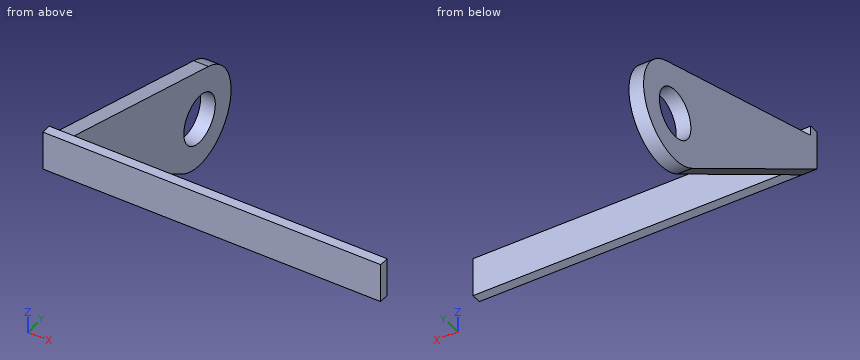
from build123d import *

# Parameters (mm, degrees)
SKETCH1_W           = 2.032
SKETCH1_H           = 0.508
BOSS_EXTRUDE1_DEPTH = 17.526
SKETCH1_3_R         = 2.54
SKETCH1_3_R_2       = 1.27
BOSS_EXTRUDE2_DEPTH = 0.762


with BuildPart() as part:
    # Sketch1 → Boss-Extrude1 (new body)
    with BuildSketch(Plane(origin=(0, 0, 0), x_dir=(0, 0, -1), z_dir=(1, 0, 0))):
        with Locations((-5.334, -11.176)):
            Rectangle(SKETCH1_W, SKETCH1_H)
    extrude(amount=BOSS_EXTRUDE1_DEPTH)

    # Sketch1_3 → Boss-Extrude2 (add)
    # profile 1 of 2: a face of its own
    with BuildSketch(Plane(origin=(0, 0, 0), x_dir=(0, 0, -1), z_dir=(1, 0, 0))):
        with BuildLine():
            Line((-4.318, -11.43), (2.137587014, -1.371977316))
            ThreePointArc((2.137587014, -1.371977316), (-1.053360752, -2.311283437), (-2.437803052, 0.713243493))
            Line((-2.437803052, 0.713243493), (-5.842, -10.922))
            Line((-5.842, -10.922), (-4.318, -10.922))
            Line((-4.318, -10.922), (-4.318, -11.43))
        make_face()
    # profile 2 of 2: a face of its own
    with BuildSketch(Plane(origin=(0, 0, 0), x_dir=(0, 0, -1), z_dir=(1, 0, 0))):
        Circle(SKETCH1_3_R)
        with Locations(Location((0, 0, 0), (0, 0, 180))):
            Circle(SKETCH1_3_R_2, mode=Mode.SUBTRACT)
    extrude(amount=BOSS_EXTRUDE2_DEPTH)


solid = part.part
Can you work these out from the model? Positions are in its coordinate system, mm. Round coordinates to 2 decimals unless told otherwise and drop trailing zeros. Order: outer loops, then holes, each group sorted by start corner. A loop starts at its lowest first (then second) coordinate and runs counter-clockwise, first axis right, second up. Notation, with made-up numbers: M -2.75,64 L 50.25,64 A7 ccw 50.25,74 Z; hole C 65.25,76.5 d7. An arc over 180 degrees is marked long. Use a Markdown table: item, result.
1) I'm going to push a flat-ended pin straight in: P1, Ø2, axis at x = 10.5, z = 5.5, coming from the +Y side. Where does the tip first touch, or does it pass through?
Geometry says:
| item | result |
|---|---|
| P1 | stops at y = -10.92 |
2) Imagine slicing it at C-C (x = 9.5). List the corners of the cut face in (y, z) for me, then the cut area to 3 significant figures.
Geometry says:
| item | result |
|---|---|
| outline | M -11.43,4.32 L -10.92,4.32 L -10.92,6.35 L -11.43,6.35 Z |
| area | 1.03 mm² |
3) Imagine slicing it at B-B (y = 1). List the corners of the cut face in (x, z) for me.
Geometry says:
| item | result |
|---|---|
| outline | M 0,-2.33 L 0.76,-2.33 L 0.76,-0.78 L 0,-0.78 Z; M 0,0.78 L 0.76,0.78 L 0.76,2.33 L 0,2.33 Z |
4) If I drill on line 1 along Y through (x, z) = (13.5, 4.75); line 2 along Y through (x, z) = (0.4, 0); line 3 along X through (y, z) = (-1.75, -1.5), over which ranges is the centre line in solid material (lowest first)?
Geometry says:
| item | result |
|---|---|
| line 1 | y = -11.43 to -10.92 |
| line 2 | y = -4.7 to -1.27, 1.27 to 2.54 |
| line 3 | x = 0 to 0.76 |
5) Imagine slicing it at A-A (z = -0.75). List the corners of the cut face in (x, y) for me, then the cut area to 3 significant figures.
Geometry says:
| item | result |
|---|---|
| outline | M 0,-3.53 L 0.76,-3.53 L 0.76,-1.02 L 0,-1.02 Z; M 0,1.02 L 0.76,1.02 L 0.76,2.43 L 0,2.43 Z |
| area | 2.98 mm² |
6) Imagine slicing it at D-D (z = 5.25). List the corners of the cut face in (x, y) for me.
Geometry says:
| item | result |
|---|---|
| outline | M 0,-11.43 L 17.53,-11.43 L 17.53,-10.92 L 0.76,-10.92 L 0.76,-8.9 L 0,-8.9 Z |
